For this review, take the finished solid that the model builds, in its own axes (mm). A direction names the side the tool comes from. Coordinates: 2 decimals unless noted, no trailing zeros. Loops run counter-clockwise (first coordinate to the right, second up) from the corner with the lowest first, then second, coordinate; pieces in that order, holes last. Notation, with made-up numbers: M 81.25,45 L 118.25,45 A14 ccw 118.25,71 Z; hole C 12.5,-35 d1. An arc over 180 degrees is marked long. Write each question's results on one line, items separated by ' | '. Start each with the question number.
```python
from build123d import *

# Parameters (mm, degrees)
F0_W     = 10
F0_H     = 5
F0_W_2   = 2
F0_H_2   = 2
F1_DEPTH = 10
F2_DEPTH = 15
F3_R     = 2


with BuildPart() as f1:
    # F0 (on Top) → F1 (new body)
    with BuildSketch(Plane.XY):
        Rectangle(F0_W, F0_H)
        Rectangle(F0_W_2, F0_H_2, mode=Mode.SUBTRACT)
        Rectangle(F0_W_2, F0_H_2)
    extrude(amount=-F1_DEPTH)

    # F0 (on Top) → F2 (join)
    with BuildSketch(Plane.XY):
        Rectangle(F0_W_2, F0_H_2)
    extrude(amount=F2_DEPTH)

    # F3
    f3_edges = [f1.edges().sort_by_distance(p)[0] for p in [
        (5, -2.5, -5),
        (-5, -2.5, -5),
        (-5, 2.5, -5),
        (5, 2.5, -5),
    ]]
    fillet(f3_edges, radius=F3_R)


solid = f1.part
```
Q1. Take a section at A-A, the plane x = -0.5. Give the boundary of the cut face in (y, z), then the cut area to 3 significant figures.
Q2. Insertion check: P1, Ø1.6, axis at x = -0.5, z = 11, coming from the -Y side; P2, Ø2, axis at y = 0, z = 10, coming from the -X side; P3, Ø1.6, axis at x = 0.5, z = 11, coming from the +Y side. Each pin has a flat end and moves straight along its axis. Give the tip position at first contact, or say it passes through.
Q3. Take a section at B-B, the plane y = 0.2. Give the boundary of the cut face in (x, z).
Q4. Take a section at C-C, the plane z = 4.5. Give the boundary of the cut face in (x, y).
Q5. Take a section at D-D, the plane x = 1.75. Give the boundary of the cut face in (y, z), then the cut area to 3 significant figures.
Q6. To check wall thickness, follow line 1 along X through (y, z) = (0.1, 14.25); line 2 along Z through (x, y) = (2, 1.7). State the ranges of each line that lie inside material, in increasing order.
Q7. For faces 1 (the face through (-1, 0, 7)), 2 (the face through (0, -1, 7)), 3 (the face through (0, 1, 7)), 4 (the face through (1, 0, 7)), list the 3-axis set-ups (+Z, -Z, +X, -X, +Y, -Y) from which the entire face can be reached by the end or side of a thin tool; tool diameter is ignored.
Results:
1) outline: M -2.5,-10 L 2.5,-10 L 2.5,0 L 1,0 L 1,15 L -1,15 L -1,0 L -2.5,0 Z | area: 80.0 mm^2
2) P1: y = -1 | P2: x = -1 | P3: y = 1
3) outline: M -5,-10 L 5,-10 L 5,0 L 1,0 L 1,15 L -1,15 L -1,0 L -5,0 Z
4) outline: M -1,-1 L 1,-1 L 1,1 L -1,1 Z
5) outline: M -2.5,-10 L 2.5,-10 L 2.5,0 L -2.5,0 Z | area: 50.0 mm^2
6) line 1: -1 to 1 | line 2: -10 to 0
7) face 1: +Z, -X, +Y, -Y | face 2: +Z, +X, -X, -Y | face 3: +Z, +X, -X, +Y | face 4: +Z, +X, +Y, -Y
